from build123d import *

# Parameters (mm, degrees)
PRISM003_DEPTH = 15
PRISM001_DEPTH = 3
PRISM_DEPTH    = 3
PRISM002_DEPTH = 15


with BuildPart() as prism003:
    # Prism003 → Prism003 (new body)
    with BuildSketch(Plane.XY):
        Polygon((101, 0), (-50.5, 87.468566), (-50.5, -87.468566), align=None)
    extrude(amount=PRISM003_DEPTH)


with BuildPart() as prism001:
    # Prism001 → Prism001 (new body)
    with BuildSketch(Plane.XY):
        Polygon((116, 0), (-58, 100.458947), (-58, -100.458947), align=None)
    extrude(amount=PRISM001_DEPTH)


with BuildPart() as cut:
    # Prism → Prism (new body)
    with BuildSketch(Plane.XY):
        Polygon((136, 0), (-68, 117.779455), (-68, -117.779455), align=None)
    extrude(amount=PRISM_DEPTH)

    # Cut: cut Prism001
    add(prism001.part, mode=Mode.SUBTRACT)


with BuildPart() as cut002:
    # Prism002 → Prism002 (new body)
    with BuildSketch(Plane.XY):
        Polygon((151, 0), (-75.5, 130.769836), (-75.5, -130.769836), align=None)
    extrude(amount=PRISM002_DEPTH)

    # Cut001: cut Cut
    add(cut.part, mode=Mode.SUBTRACT)

    # Cut002: cut Prism003
    add(prism003.part, mode=Mode.SUBTRACT)


solid = cut002.part
The listing builds one solid part. Answer for the finished solid, in the listing's coordinates (mm). A direction names the side the tool comes from. Round coordinates to 2 decimals unless told otherwise and drop trailing zeros. Order: outer loops, then holes, each group sorted by start corner. A loop starts at its lowest first (then second) coordinate and runs counter-clockwise, first axis right, second up. Notation, with made-up numbers: M 68,63 L 113,63 A18 ccw 113,90 Z; hole C 3.25,34 d1. An arc over 180 degrees is marked long. Answer in a Markdown table with one row per item. Add a question column.
1) The part is cut by section D-D on x = 130.5. Determine the outline of the cut face in (y, z), plus the area to 3 significant figures.
2) Consider line 1 along Y through (x, z) = (-49.5, 0.5); line 2 along Y through (x, z) = (2.5, 1); line 3 along Z through (x, y) = (-3, 69). Determine where each line is inside the solid, lowest interval first. Write a range as from..to.
3) The part is cut by section B-B on z = 7. Determine the outline of the cut face in (x, y), plus the area to 3 significant figures.
4) Which of the six approach directions +Z, -Z, +X, -X, +Y, -Y give full straight-line access (tool end or side, diameter ignored) to faces 1 (the face through (29, 45, 0)), 2 (the face through (24.19, -44.347, 7.395)), 3 (the face through (30.218, 49.526, 1.479))?
5) The part is cut by section C-C on y = -84.5. Determine the outline of the cut face in (x, z), plus the area to 4 significant figures.
6) The part is cut by section A-A on x = 18. Determine the outline of the cut face in (y, z), plus the area to 3 significant figures.
7) Flat-ended cylindrical pins translate along their axes: pin 1 Ø2.5 at (y, z) = (-54.5, 1.5) entering from +X; pin 2 Ø2 at (y, z) = (5.5, 9) entering from +X; pin 3 Ø8 at (x, y) = (55, 61) entering from +Z; pin 4 Ø1.5 at (x, z) = (42, 8.5) entering from -Y. Find the tip coordinate at first contact, or state that the pin passes through.
8) Determine the mould class of faces 4 (the face through (26, 53, 3)), 5 (the face through (-50.5, 1, 7)), 6 (the face through (39.335, 64.47, 7.395)), 7 (the face through (20, -48, 15)) for opening direction X: pulls with the +X half, pulls with the -X half, needs draft (parallel to the pull), parting line crosses it, or undercut.
Findings below:
| question | item | result |
|---|---|---|
| 1 | outline | M -11.84,0 L -3.18,0 L -3.18,3 L 3.18,3 L 3.18,0 L 11.84,0 L 11.84,15 L -11.84,15 Z |
| 1 | area | 336 mm² |
| 2 | line 1 | y = -115.76..-107.1, -95.55..-86.89, 86.89..95.55, 107.1..115.76 |
| 2 | line 2 | y = -85.74..-77.08, -65.53..-56.87, 56.87..65.53, 77.08..85.74 |
| 2 | line 3 | z = 3..15 |
| 3 | outline | M -75.5,-130.77 L 151,0 L -75.5,130.77 Z; hole M -50.5,-87.47 L 101,0 L -50.5,87.47 Z |
| 3 | area | 16,400 mm² |
| 4 | face 1 | -Z, +X, -X, +Y, -Y |
| 4 | face 2 | +Z, -Z |
| 4 | face 3 | -Z |
| 5 | outline | M -75.5,0 L -68,0 L -68,3 L -58,3 L -58,0 L -50.5,0 L -50.5,15 L -75.5,15 Z; M -45.36,0 L -30.36,0 L -30.36,3 L -10.36,3 L -10.36,0 L 4.64,0 L 4.64,15 L -45.36,15 Z |
| 5 | area | 1,035 mm² |
| 6 | outline | M -76.79,0 L -68.13,0 L -68.13,3 L -56.58,3 L -56.58,0 L -47.92,0 L -47.92,15 L -76.79,15 Z; M 47.92,0 L 56.58,0 L 56.58,3 L 68.13,3 L 68.13,0 L 76.79,0 L 76.79,15 L 47.92,15 Z |
| 6 | area | 797 mm² |
| 7 | pin 1 | stops at x = 58.77 |
| 7 | pin 2 | stops at x = 143.21 |
| 7 | pin 3 | passes through |
| 7 | pin 4 | stops at y = -63.36 |
| 8 | face 4 | undercut |
| 8 | face 5 | undercut |
| 8 | face 6 | pulls with the +X half |
| 8 | face 7 | needs draft |
